CAD build for the part. Positions are in the model's coordinates, mm. A direction names the side the tool comes from. Coordinates: 2 decimals unless noted, no trailing zeros. Write each loop counter-clockwise with the first axis right and the second up, starting at its lowest first coordinate (ties: lowest second). Pieces come first, ordered by that corner, then holes. Notation, with made-up numbers: (-35, 38.25) -> (16, 38.25) arc R28 cw to (16, 63.25) -> close; hole circle Ø10 at (31.5, 26.5). An arc over 180 degrees is marked (long way). Answer as CSV lines item,"result".
```python
from build123d import *

# Parameters (mm, degrees)
F0_R     = 76.2
F1_DEPTH = 152.4
F1_TAPER = 10
F2_R     = 31.75
F3_DEPTH = 25.4
F4_R     = 6.35
F5_DEPTH = 76.2
F6_W     = 19.05
F6_H     = 19.05
F6_R     = 6.35
F7_DEPTH = 19.05
F8_R     = 6.35
F9_DEPTH = 304.8


with BuildPart() as f1:
    # F0 (on Top) → F1 (new body)
    with BuildSketch(Plane.XY):
        Circle(F0_R)
    extrude(amount=F1_DEPTH, taper=F1_TAPER)

    # F2 (on face) → F3 (join)
    with BuildSketch(Plane.XY.offset(152.4)):
        Circle(F2_R)
    extrude(amount=F3_DEPTH)

    # F4 (on face) → F5 (join)
    with BuildSketch(Plane.XY.offset(177.8)):
        Circle(F4_R)
    extrude(amount=F5_DEPTH)

    # F6 (on face) → F7 (join)
    with BuildSketch(Plane.XY.offset(254)):
        Rectangle(F6_W, F6_H)
        Circle(F6_R, mode=Mode.SUBTRACT)
        Circle(F6_R)
    extrude(amount=F7_DEPTH)

    # F8 (on face) → F9 (join)
    with BuildSketch(Plane.YZ.offset(9.525)):
        with Locations((0, 263.525)):
            Circle(F8_R)
    extrude(amount=F9_DEPTH)


solid = f1.part
```
Item 1: 3-axis set-ups, long thin cutter, end or side, ignore diameter. For faces 4 (the cylindrical face through (159.79, -0.83, 269.82)), 5 (the cylindrical face through (-1.38, -6.2, 215.37)), 6 (the flat face through (0, -9.525, 263)): which of +Z, -Z, +X, -X, +Y, -Y reach the whole face in a straight line?
Answer below:
face 4,"+X"
face 5,"none"
face 6,"+Z, +X, -X, -Y"
Item 2: Saw through at D-D on z = 124. Give the cut face in (x, y), and give its area (3 significant figures).
Answer below:
outline,"circle Ø108.67 at (0, 0)"
area,"9,280 mm2"
Item 3: Saw through at A-A on y = 0. Give the cut face in (x, z) (3 decimals).
Answer below:
outline,"(-76.2, 0) -> (76.2, 0) -> (49.328, 152.4) -> (31.75, 152.4) -> (31.75, 177.8) -> (6.35, 177.8) -> (6.35, 254) -> (9.525, 254) -> (9.525, 257.175) -> (314.325, 257.175) -> (314.325, 269.875) -> (9.525, 269.875) -> (9.525, 273.05) -> (-9.525, 273.05) -> (-9.525, 254) -> (-6.35, 254) -> (-6.35, 177.8) -> (-31.75, 177.8) -> (-31.75, 152.4) -> (-49.328, 152.4) -> close"
Item 4: Saw through at B-B on x = 0. Give the cut face in (y, z) (3 decimals).
Answer below:
outline,"(-76.2, 0) -> (76.2, 0) -> (49.328, 152.4) -> (31.75, 152.4) -> (31.75, 177.8) -> (6.35, 177.8) -> (6.35, 254) -> (9.525, 254) -> (9.525, 273.05) -> (-9.525, 273.05) -> (-9.525, 254) -> (-6.35, 254) -> (-6.35, 177.8) -> (-31.75, 177.8) -> (-31.75, 152.4) -> (-49.328, 152.4) -> close"
Item 5: Saw through at C-C on z = 196. Give the cut face in (x, y).
Answer below:
outline,"circle Ø12.7 at (0, 0)"
Item 6: Flat gauge pins, fed straight in: pin 1 (2 mm diameter, centred on y = -32, z = 64.5, fed in from -X); pin 2 (5.5 mm diameter, centred on y = -4.5, z = 263.5, fed in from -X) (3 decimals); pin 3 (5 mm diameter, centred on x = 229, y = 0.5, fed in from +Z) (3 decimals). Where does each tip first touch, or does it go through?
Answer below:
pin 1,"stops at x = -56.97"
pin 2,"stops at x = -9.525"
pin 3,"stops at z = 269.875"
Item 7: Wall check: line 1 (Z direction, x = 7, y = -39); line 2 (X direction, y = -19, z = 54); line 3 (Y direction, x = -36.5, z = 96.5). Give the ranges that are in metal, low to high. Write a range as from..to.
Answer below:
line 1,"z = 0..152.4"
line 2,"x = -63.91..63.91"
line 3,"y = -46.59..46.59"
Item 8: Two-plate mould, pull along Z, no slides. Class faces 1 (the flat face through (-0.1, 6.5, 254)), 2 (the flat face through (-9.525, 0, 263)), 3 (the flat face through (0, 0, 273.05)): pulls with the +Z half, pulls with the -Z half, needs draft (parallel to the pull), parting line crosses it, or undercut.
Answer below:
face 1,"undercut"
face 2,"needs draft"
face 3,"pulls with the +Z half"
